```python
from build123d import *

# Parameters (mm, degrees)
SKETCH1_W                        = 110
SKETCH1_H                        = 80
BOSS_EXTRUDE1_DEPTH              = 3
SKETCH2_W                        = 110
SKETCH2_H                        = 6
BOSS_EXTRUDE2_DEPTH              = 8
F_1_8_27_NPSM_TAPPED_HOLE1_D     = 5
F_1_8_27_NPSM_TAPPED_HOLE1_DEPTH = 6
F_1_8_27_NPSM_TAPPED_HOLE1_TIP   = 1.502151548
FILLET1_R                        = 3
CUT_EXTRUDE1_DEPTH               = 8
LPATTERN1_COUNT                  = 6
LPATTERN1_PITCH                  = 12.5
CUT_EXTRUDE2_DEPTH               = 8
FILLET2_R                        = 3
CHAMFER1_SIZE                    = 1


with BuildPart() as part:
    # Sketch1 → Boss-Extrude1 (new body)
    with BuildSketch(Plane(origin=(0, 0, 0), x_dir=(1, 0, 0), z_dir=(0, 1, 0))):
        Rectangle(SKETCH1_W, SKETCH1_H)
    extrude(amount=BOSS_EXTRUDE1_DEPTH)

    # Sketch2 → Boss-Extrude2 (add)
    with BuildSketch(Plane(origin=(0, 3, 0), x_dir=(1, 0, 0), z_dir=(0, 1, 0))):
        with Locations((0, -37)):
            Rectangle(SKETCH2_W, SKETCH2_H)
    extrude(amount=BOSS_EXTRUDE2_DEPTH)

    # 1/8-27 NPSM Tapped Hole1
    with Locations(Plane.XY.offset(40)):
        with Locations((-35, 4.5), (35, 4.5)):
            Hole(F_1_8_27_NPSM_TAPPED_HOLE1_D / 2, depth=F_1_8_27_NPSM_TAPPED_HOLE1_DEPTH)
            with Locations((0, 0, -(F_1_8_27_NPSM_TAPPED_HOLE1_DEPTH + F_1_8_27_NPSM_TAPPED_HOLE1_TIP / 2))):  # 118° drill point
                Cone(0, F_1_8_27_NPSM_TAPPED_HOLE1_D / 2, F_1_8_27_NPSM_TAPPED_HOLE1_TIP, mode=Mode.SUBTRACT)

    # Fillet1
    # the kernel refuses this fillet: 3 mm, written as the material it adds along each edge
    with BuildSketch(Plane(origin=(55, 3, 34), x_dir=(0, 0, -1), z_dir=(-1, 0, 0))) as fillet1_piece_1_section:
        with BuildLine():
            CenterArc((FILLET1_R, -FILLET1_R), FILLET1_R, 90, 90)
            Line((0, -FILLET1_R), (0, 0))
            Line((0, 0), (FILLET1_R, 0))
        make_face()
    fillet1_piece_1 = extrude(amount=25.5, mode=Mode.PRIVATE)
    fillet1_piece_1 = fillet1_piece_1 - Plane(origin=(35, 4.5, 33.326842019), x_dir=(-1, 0, 0), z_dir=(0, 0, -1)) * Cylinder(2.5, 64, mode=Mode.PRIVATE)
    add(fillet1_piece_1)
    with BuildSketch(Plane(origin=(40.5, 3, 34), x_dir=(0, 0, -1), z_dir=(-1, 0, 0))) as fillet1_piece_2_section:
        with BuildLine():
            CenterArc((FILLET1_R, -FILLET1_R), FILLET1_R, 90, 90)
            Line((0, -FILLET1_R), (0, 0))
            Line((0, 0), (FILLET1_R, 0))
        make_face()
    fillet1_piece_2 = extrude(amount=81, mode=Mode.PRIVATE)
    fillet1_piece_2 = fillet1_piece_2 - Plane(origin=(35, 4.5, 33.313079734), x_dir=(-1, 0, 0), z_dir=(0, 0, -1)) * Cylinder(2.5, 175, mode=Mode.PRIVATE)
    fillet1_piece_2 = fillet1_piece_2 - Plane(origin=(-35, 4.5, 33.313079734), x_dir=(-1, 0, 0), z_dir=(0, 0, -1)) * Cylinder(2.5, 175, mode=Mode.PRIVATE)
    add(fillet1_piece_2)
    with BuildSketch(Plane(origin=(-29.5, 3, 34), x_dir=(0, 0, -1), z_dir=(-1, 0, 0))) as fillet1_piece_3_section:
        with BuildLine():
            CenterArc((FILLET1_R, -FILLET1_R), FILLET1_R, 90, 90)
            Line((0, -FILLET1_R), (0, 0))
            Line((0, 0), (FILLET1_R, 0))
        make_face()
    fillet1_piece_3 = extrude(amount=25.5, mode=Mode.PRIVATE)
    fillet1_piece_3 = fillet1_piece_3 - Plane(origin=(-35, 4.5, 33.313079734), x_dir=(-1, 0, 0), z_dir=(0, 0, -1)) * Cylinder(2.5, 63, mode=Mode.PRIVATE)
    add(fillet1_piece_3)
    # the kernel refuses this fillet: 3 mm, written as the material it takes off along each edge
    with BuildSketch(Plane(origin=(62.5, 11, 34), x_dir=(0, -1, 0), z_dir=(-1, 0, 0))) as fillet1_2_piece_1:
        with BuildLine():
            CenterArc((FILLET1_R, FILLET1_R), FILLET1_R, 180, 90)
            Line((0, FILLET1_R), (0, 0))
            Line((0, 0), (FILLET1_R, 0))
        make_face()
    extrude(amount=125, mode=Mode.SUBTRACT)

    # Sketch6 → Cut-Extrude1 (cut)
    with BuildSketch(Plane(origin=(0, 3, 0), x_dir=(1, 0, 0), z_dir=(0, 1, 0))):
        with BuildLine():
            Line((-41.150032335, -24), (-21.150032335, -24))
            ThreePointArc((-21.150032335, -24), (-19.400032335, -25.75), (-21.150032335, -27.5))
            Line((-21.150032335, -27.5), (-41.150032335, -27.5))
            ThreePointArc((-41.150032335, -27.5), (-42.900032335, -25.75), (-41.150032335, -24))
        make_face()
        with BuildLine():
            Line((41.150032335, -24), (21.150032335, -24))
            ThreePointArc((21.150032335, -24), (19.400032335, -25.75), (21.150032335, -27.5))
            Line((21.150032335, -27.5), (41.150032335, -27.5))
            ThreePointArc((41.150032335, -27.5), (42.900032335, -25.75), (41.150032335, -24))
        make_face()
    cut_extrude1 = extrude(amount=-CUT_EXTRUDE1_DEPTH, mode=Mode.SUBTRACT)

    # LPattern1: Cut-Extrude1 ×6
    with Locations(*[(0, 0, -i * LPATTERN1_PITCH) for i in range(1, LPATTERN1_COUNT)]):
        add(cut_extrude1, mode=Mode.SUBTRACT)

    # Sketch7 → Cut-Extrude2 (cut)
    with BuildSketch(Plane(origin=(0, 3, 0), x_dir=(1, 0, 0), z_dir=(0, 1, 0))):
        with BuildLine():
            Line((-13.750692764, -24.031822976), (-13.750692764, 33.113913187))
            ThreePointArc((-13.750692764, 33.113913187), (-9.15862468, 37.705981272), (-4.566556595, 33.113913187))
            Line((-4.566556595, 33.113913187), (-4.566556595, -24.031822976))
            ThreePointArc((-4.566556595, -24.031822976), (-9.15862468, -28.62389106), (-13.750692764, -24.031822976))
        make_face()
        with BuildLine():
            Line((13.750692764, -24.031822976), (13.750692764, 33.113913187))
            ThreePointArc((13.750692764, 33.113913187), (9.15862468, 37.705981272), (4.566556595, 33.113913187))
            Line((4.566556595, 33.113913187), (4.566556595, -24.031822976))
            ThreePointArc((4.566556595, -24.031822976), (9.15862468, -28.62389106), (13.750692764, -24.031822976))
        make_face()
    extrude(amount=-CUT_EXTRUDE2_DEPTH, mode=Mode.SUBTRACT)

    # Fillet2
    fillet2_edges = [part.edges().sort_by_distance(p)[0] for p in [
        (-55, 5.5, 40),
        (55, 5.5, 40),
        (55, 1.5, -40),
        (-55, 1.5, -40),
    ]]
    fillet(fillet2_edges, radius=FILLET2_R)

    # Chamfer1
    chamfer1_edges = [part.edges().sort_by_distance(p)[0] for p in [
        (-42.900032335, 3, 25.75),
        (-31.150032335, 3, 27.5),
        (-19.400032335, 3, 25.75),
        (-31.150032335, 3, 24),
        (42.900032335, 3, 25.75),
        (31.150032335, 3, 24),
        (19.400032335, 3, 25.75),
        (31.150032335, 3, 27.5),
        (-42.900032335, 3, 13.25),
        (-31.150032335, 3, 15),
        (-19.400032335, 3, 13.25),
        (-31.150032335, 3, 11.5),
        (-42.900032335, 3, 0.75),
        (-31.150032335, 3, -1),
        (-19.400032335, 3, 0.75),
        (-31.150032335, 3, 2.5),
        (-42.900032335, 3, -11.75),
        (-31.150032335, 3, -13.5),
        (-19.400032335, 3, -11.75),
        (-31.150032335, 3, -10),
        (-42.900032335, 3, -24.25),
        (-31.150032335, 3, -26),
        (-19.400032335, 3, -24.25),
        (-31.150032335, 3, -22.5),
        (-42.900032335, 3, -36.75),
        (-31.150032335, 3, -38.5),
        (-19.400032335, 3, -36.75),
        (-31.150032335, 3, -35),
        (42.900032335, 3, 13.25),
        (31.150032335, 3, 11.5),
        (19.400032335, 3, 13.25),
        (31.150032335, 3, 15),
        (42.900032335, 3, 0.75),
        (31.150032335, 3, 2.5),
        (19.400032335, 3, 0.75),
        (31.150032335, 3, -1),
        (42.900032335, 3, -11.75),
        (31.150032335, 3, -10),
        (19.400032335, 3, -11.75),
        (31.150032335, 3, -13.5),
        (42.900032335, 3, -24.25),
        (31.150032335, 3, -22.5),
        (19.400032335, 3, -24.25),
        (31.150032335, 3, -26),
        (42.900032335, 3, -36.75),
        (31.150032335, 3, -35),
        (19.400032335, 3, -36.75),
        (31.150032335, 3, -38.5),
        (-9.15862468, 3, 28.62389106),
        (-4.566556595, 3, -4.541045106),
        (-9.15862468, 3, -37.705981272),
        (-13.750692764, 3, -4.541045106),
        (9.15862468, 3, 28.62389106),
        (13.750692764, 3, -4.541045106),
        (9.15862468, 3, -37.705981272),
        (4.566556595, 3, -4.541045106),
    ]]
    chamfer(chamfer1_edges, length=CHAMFER1_SIZE)


solid = part.part
```
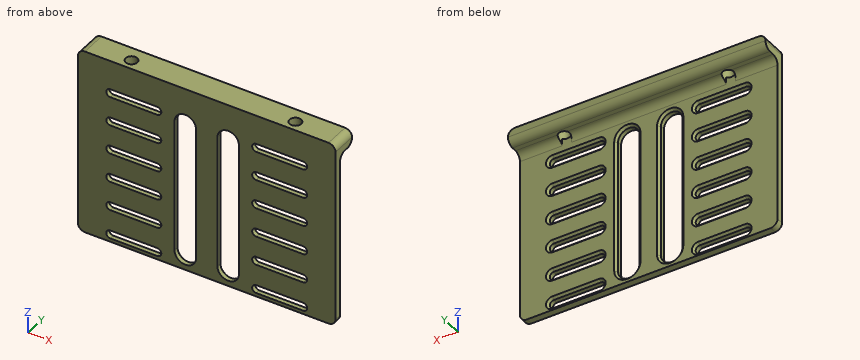
Model file for the job. Use its own axes, mm. Coordinates: 2 decimals unless noted, no trailing zeros. Loops run counter-clockwise (first coordinate to the right, second up) from the corner with the lowest first, then second, coordinate; pieces in that order, holes last. Notation, with made-up numbers: (17, -33.75) - (65, -33.75) arc R23 cw to (65, -12.75) - close; hole circle Ø3 at (6.25, 30). An arc over 180 degrees is marked (long way). Answer as a JSON object with one key per item and string values. Group by question number.
(1) Cut at A-A (z = 0.75). Give the cut face in (x, y).
(2) Flat gauge pin, fed straight in: pin 1 (12 mm diameter, centred on x = -36, z = -1.5, fed in from +Y). Where does the tip first touch, or does it go through?
(3) Probe line 1 along X through (y, z) = (4.5, 35); line 2 along X through (y, z) = (0.75, -27); line 3 along Z through (x, y) = (-45, 7.5). List the from-to ranges inside material, lowest first.
(4) Cut at B-B (x = -40). State how many separate pieces and enclosed holes the cut face has, then the cut area to 3 significant figures.
Geometry says:
{
 "1": {"outline": "(-55, 0) - (-42.9, 0) - (-42.9, 2) - (-43.9, 3) - (-55, 3) - close; (-19.4, 0) - (-13.75, 0) - (-13.75, 2) - (-14.75, 3) - (-18.4, 3) - (-19.4, 2) - close; (-4.57, 0) - (4.57, 0) - (4.57, 2) - (3.57, 3) - (-3.57, 3) - (-4.57, 2) - close; (13.75, 0) - (19.4, 0) - (19.4, 2) - (18.4, 3) - (14.75, 3) - (13.75, 2) - close; (42.9, 0) - (55, 0) - (55, 3) - (43.9, 3) - (42.9, 2) - close"},
 "2": {"pin 1": "stops at y = 3"},
 "3": {"line 1": "x = -55 to -37.5, -32.5 to 32.5, 37.5 to 55", "line 2": "x = -55 to -13.75, -4.57 to 4.57, 13.75 to 55", "line 3": "z = 34 to 40"},
 "4": {"separate pieces": "7", "enclosed holes": "0", "area": "219 mm^2"}
}
